Build history of the part. All positions in model axes, mm. Face numbers are marked on the shaded views. A direction names the side the tool comes from. Coordinates: 2 decimals unless noted, no trailing zeros. Write each loop counter-clockwise with the first axis right and the second up, starting at its lowest first coordinate (ties: lowest second). Pieces come first, ordered by that corner, then holes.
from build123d import *

# Parameters (mm, degrees)
SKETCH1_W           = 140
SKETCH1_H           = 130
BOSS_EXTRUDE1_DEPTH = 52
SHELL1_T            = -3
SKETCH2_R           = 3.5
SKETCH2_R_2         = 2
SKETCH2_R_3         = 1.1
CUT_EXTRUDE1_DEPTH  = 137
SKETCH3_R           = 1.1
CUT_EXTRUDE2_DEPTH  = 3
CUT_EXTRUDE4_DEPTH  = 3
SKETCH7_R           = 4.775
CUT_EXTRUDE5_DEPTH  = 2
CIRPATTERN5_COUNT   = 2
SKETCH8_W           = 12
SKETCH8_H           = 15
BOSS_EXTRUDE2_DEPTH = 2
SKETCH11_R          = 1.5
CUT_EXTRUDE7_DEPTH  = 118.473401245
FILLET1_R           = 3
FILLET2_R           = 3
CHAMFER1_SIZE       = 3
SKETCH12_R          = 8
CUT_EXTRUDE8_DEPTH  = 10


with BuildPart() as part:
    # Sketch1 → Boss-Extrude1 (new body)
    with BuildSketch(Plane(origin=(0, 0, 0), x_dir=(1, 0, 0), z_dir=(0, 1, 0))):
        Rectangle(SKETCH1_W, SKETCH1_H)
    extrude(amount=BOSS_EXTRUDE1_DEPTH)

    # Shell1
    shell1_openings = [part.faces().sort_by_distance(p)[0] for p in [
        (0, 52, 0),
    ]]
    offset(amount=SHELL1_T, openings=shell1_openings, kind=Kind.INTERSECTION)

    # Sketch2 → Cut-Extrude1 (cut)
    with BuildSketch(Plane(origin=(70, 0, 0), x_dir=(0, 0, -1), z_dir=(1, 0, 0))):
        with Locations((21.837588157, 25.5)):
            Circle(SKETCH2_R)
        with Locations((32.837588157, 25.5)):
            Circle(SKETCH2_R_2)
        with Locations((12.837588157, 34.5)):
            Circle(SKETCH2_R_3)
        with Locations((12.837588157, 16.5)):
            Circle(SKETCH2_R_3)
    cut_extrude1 = extrude(amount=-CUT_EXTRUDE1_DEPTH, mode=Mode.SUBTRACT)

    # Mirror1: Cut-Extrude1 across plane
    add(cut_extrude1.mirror(Plane(origin=(0, 0, 0), x_dir=(0, 0, 1), z_dir=(1, 0, 0))), mode=Mode.SUBTRACT)

    # Sketch3 → Cut-Extrude2 (cut)
    with BuildSketch(Plane(origin=(0, 3, 0), x_dir=(1, 0, 0), z_dir=(0, 1, 0))):
        with Locations(Location((-7, -59, 0), (0, 0, 270))):
            Circle(SKETCH3_R)
        with Locations(Location((7, -59, 0), (0, 0, 270))):
            Circle(SKETCH3_R)
    extrude(amount=-CUT_EXTRUDE2_DEPTH, mode=Mode.SUBTRACT)

    # Sketch6 → Cut-Extrude4 (cut)
    with BuildSketch(Plane(origin=(0, 0, 62), x_dir=(-1, 0, 0), z_dir=(0, 0, -1))):
        with BuildLine():
            Line((55, 4), (49, 4))
            ThreePointArc((49, 4), (47, 6), (49, 8))
            Line((49, 8), (55, 8))
            ThreePointArc((55, 8), (57, 6), (55, 4))
        make_face()
    extrude(amount=-CUT_EXTRUDE4_DEPTH, mode=Mode.SUBTRACT)

    # Sketch7 → Cut-Extrude5 (cut)
    with BuildSketch(Plane(origin=(-67, 0, 0), x_dir=(0, 0, -1), z_dir=(1, 0, 0))):
        with Locations((50, 43.5)):
            Circle(SKETCH7_R)
    cut_extrude5 = extrude(amount=-CUT_EXTRUDE5_DEPTH, mode=Mode.SUBTRACT)

    # CirPattern5: Cut-Extrude5 ×2 about axis
    cirpattern5_axis = Axis((0, 54.6, 0), (0, -1, 0))
    for i in range(1, CIRPATTERN5_COUNT):
        add(cut_extrude5.rotate(cirpattern5_axis, i * 360 / CIRPATTERN5_COUNT), mode=Mode.SUBTRACT)

    # Sketch8 → Boss-Extrude2 (add)
    with BuildSketch(Plane(origin=(0, 0, 0), x_dir=(1, 0, 0), z_dir=(0, 1, 0))):
        with Locations((-37.75, -72.5)):
            Rectangle(SKETCH8_W, SKETCH8_H)
        with Locations((28.25, -72.5)):
            Rectangle(SKETCH8_W, SKETCH8_H)
    extrude(amount=BOSS_EXTRUDE2_DEPTH)

    # Sketch11 → Cut-Extrude7 (cut, through all)
    with BuildSketch(Plane(origin=(0, 2, 0), x_dir=(1, 0, 0), z_dir=(0, 1, 0))):
        with Locations(Location((-39.25, -76, 0), (0, 0, 270))):
            Circle(SKETCH11_R)
        with Locations(Location((30.25, -76, 0), (0, 0, 270))):
            Circle(SKETCH11_R)
    extrude(amount=-CUT_EXTRUDE7_DEPTH, mode=Mode.SUBTRACT)

    # Fillet1
    fillet1_edges = [part.edges().sort_by_distance(p)[0] for p in [
        (-43.75, 1, 65),
        (-43.75, 1, 80),
        (34.25, 1, 80),
        (34.25, 1, 65),
    ]]
    fillet(fillet1_edges, radius=FILLET1_R)

    # Fillet2
    fillet2_edges = [part.edges().sort_by_distance(p)[0] for p in [
        (-31.75, 1, 80),
        (-31.75, 1, 65),
        (22.25, 1, 80),
        (22.25, 1, 65),
    ]]
    fillet(fillet2_edges, radius=FILLET2_R)

    # Chamfer1
    chamfer1_edges = [part.edges().sort_by_distance(p)[0] for p in [
        (28.25, 2, 65),
        (-37.75, 2, 65),
    ]]
    chamfer(chamfer1_edges, length=CHAMFER1_SIZE)

    # Sketch12 → Cut-Extrude8 (cut)
    with BuildSketch(Plane.XY.offset(65)):
        with Locations((-13, 15.5)):
            Circle(SKETCH12_R)
        with Locations((13, 15.5)):
            Circle(SKETCH12_R)
        with BuildLine():
            Line((-3.1, 9.5), (3.1, 9.5))
            ThreePointArc((3.1, 9.5), (4.85, 7.75), (3.1, 6))
            Line((3.1, 6), (-3.1, 6))
            ThreePointArc((-3.1, 6), (-4.85, 7.75), (-3.1, 9.5))
        make_face()
    extrude(amount=-CUT_EXTRUDE8_DEPTH, mode=Mode.SUBTRACT)


solid = part.part
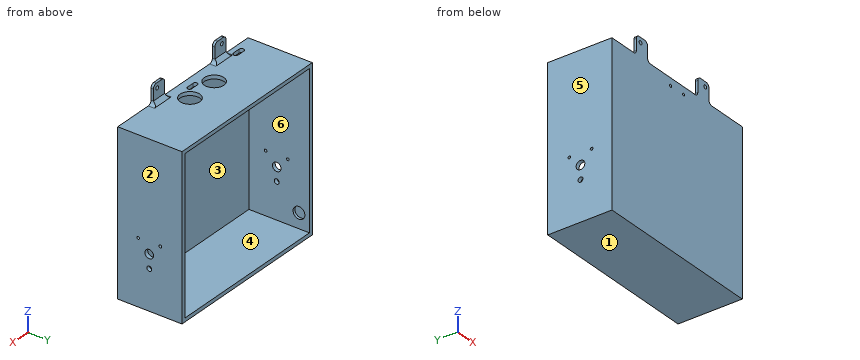
(1) Flat gauge pins, fed straight in: P1, Ø2.5, axis at x = 30.25, z = 76, coming from the +Y side; P2, Ø5, axis at x = 36, z = -6, coming from the +Y side; P3, Ø4, axis at x = -24.5, y = 42.5, coming from the +Z side; P4, Ø6, axis at x = 26, z = 73, coming from the +Y side. Where does each tip first touch, or does it go through?
(2) Two-plate mould, pull along X, no slides. Class the marked faces 1, 2, 3 and 4: pulls with the +X half, pulls with the -X half, needs draft (parallel to the pull), parting line crosses it, or undercut.
(3) Probe L1, parallel to X at y = 2, z = 59; L2, parallel to Z at x = -67.9, y = 25.5; L3, parallel to X at y = 34.5, z = 34.5. List the from-to ranges inside material, lowest first.
(4) 3-axis set-ups, long thin cutter, end or side, ignore diameter. For the marked faces 5 and 6: which of +Z, -Z, +X, -X, +Y, -Y reach the whole face in a straight line?
(5) Slice it at D-D, the plane x = -26. List the corners of the cut face in (y, z), and give its area (3 significant figures).
(6) Slice it at B-B, the plane z = -3.5. List the corners of the cut face in (x, y).
(7) Slice it at C-C, the plane x = -12. List the corners of the cut face in (y, z).
(8) Slice it at A-A, the plane y = 31.5. List the corners of the cut face in (x, z), and give its area (3 significant figures).
Results:
1. P1: passes through
1. P2: stops at y = 3
1. P3: stops at z = 65
1. P4: stops at y = 2
2. face 1: needs draft
2. face 2: pulls with the +X half
2. face 3: undercut
2. face 4: undercut
3. L1: x = -70 to -8.1, -5.9 to 5.9, 8.1 to 70
3. L2: z = -65 to -34.84, -30.84 to -25.34, -18.34 to 65
3. L3: x = -70 to -67, 67 to 70
4. face 5: +Z, -Z, -X, +Y, -Y
4. face 6: +Y
5. outline: (0, -65) - (52, -65) - (52, -62) - (3, -62) - (3, 62) - (52, 62) - (52, 65) - (0, 65) - close
5. area: 684 mm2
6. outline: (-70, 0) - (70, 0) - (70, 52) - (67, 52) - (67, 3) - (-67, 3) - (-67, 52) - (-70, 52) - close
7. outline: (0, -65) - (52, -65) - (52, -62) - (3, -62) - (3, 62) - (7.56, 62) - (7.56, 65) - (0, 65) - close; (23.44, 62) - (52, 62) - (52, 65) - (23.44, 65) - close
8. outline: (-70, -65) - (70, -65) - (70, 65) - (-70, 65) - close; hole (-67, -62) - (67, -62) - (67, 62) - (-67, 62) - close
8. area: 1,580 mm2
